Read the model definition and answer for the solid it produces. Units are mm, in the model's axes. Face numbers are marked on the shaded views. A direction names the side the tool comes from. Coordinates: 2 decimals unless noted, no trailing zeros. Loops run counter-clockwise (first coordinate to the right, second up) from the corner with the lowest first, then second, coordinate; pieces in that order, holes last. Notation, with made-up numbers: (63.25, 68.5) -> (77.25, 68.5) arc R28 ccw to (77.25, 86.5) -> close; hole circle Ø2 at (-35, 22.25). An arc over 180 degrees is marked (long way). Answer in a Markdown table with one row per item.
```python
from build123d import *

# Parameters (mm, degrees)
F0_W     = 30
F0_H     = 30
F1_DEPTH = 30
F2_SIZE  = 3.1
F3_R     = 10
F4_DEPTH = 32.5
F6_DEPTH = 1
F8_DEPTH = 1


with BuildPart() as f1:
    # F0 (on Top) → F1 (new body)
    with BuildSketch(Plane.XY):
        Rectangle(F0_W, F0_H)
    extrude(amount=F1_DEPTH)

    # F2
    f2_edges = [f1.edges().sort_by_distance(p)[0] for p in [
        (0, -15, 30),
        (15, 0, 30),
        (15, -15, 15),
        (-15, 0, 0),
        (0, 15, 0),
        (-15, 15, 15),
        (0, 15, 30),
        (15, 15, 15),
        (-15, -15, 15),
        (0, -15, 0),
        (15, 0, 0),
        (-15, 0, 30),
    ]]
    chamfer(f2_edges, length=F2_SIZE)

    # F3 (on Top) → F4 (join)
    with BuildSketch(Plane.XY):
        Circle(F3_R)
    extrude(amount=F4_DEPTH)

    # F5 (on face) → F6 (join)
    with BuildSketch(Plane.XZ.offset(15)):
        Polygon((-9.9, 26.9), (-9.9, 3.1), (-4.9, 3.1), align=None)
        Polygon((9.9, 3.1), (9.9, 26.9), (4.9, 26.9), align=None)
        Polygon((-7.9, 26.9), (-2.9, 3.1), (7.9, 3.1), (2.9, 26.9), align=None)
    extrude(amount=F6_DEPTH)

    # F7 (on face) → F8 (join)
    with BuildSketch(Plane(origin=(0, 15, 0), x_dir=(-1, 0, 0), z_dir=(0, 1, 0))):
        Polygon((-2.9, 26.9), (-7.9, 3.1), (2.9, 3.1), (7.9, 26.9), align=None)
        Polygon((9.9, 26.9), (4.9, 3.1), (9.9, 3.1), align=None)
        Polygon((-4.9, 26.9), (-9.9, 26.9), (-9.9, 3.1), align=None)
    extrude(amount=F8_DEPTH)


solid = f1.part
```
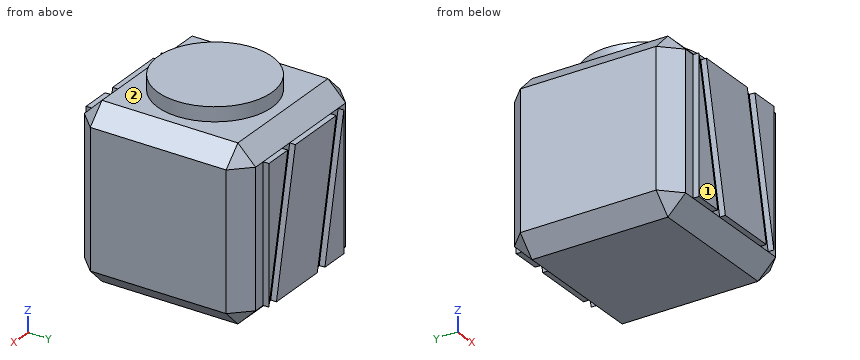
1. A cutting plane is placed at D-D on x = 6.75. Give the vertices of the cut face in (y, z).
A:
| item | result |
|---|---|
| outline | (-16, 3.1) -> (-15, 3.1) -> (-11.9, 0) -> (11.9, 0) -> (15, 3.1) -> (16, 3.1) -> (16, 8.57) -> (15, 8.57) -> (15, 18.09) -> (16, 18.09) -> (16, 26.9) -> (15, 26.9) -> (11.9, 30) -> (7.38, 30) -> (7.38, 32.5) -> (-7.38, 32.5) -> (-7.38, 30) -> (-11.9, 30) -> (-15, 26.9) -> (-16, 26.9) -> (-16, 18.09) -> (-15, 18.09) -> (-15, 8.57) -> (-16, 8.57) -> close |
2. A tool of negligible diameter and unlimited length cuts with its end or side. For the marked faces 1 and 2, from which of +Z, -Z, +X, -X, +Y, -Y can it reach the whole face along a straight path? Write none if from no direction.
A:
| item | result |
|---|---|
| face 1 | +Z, -Z, +X, -X, -Y |
| face 2 | +Z |
3. A cutting plane is placed at A-A on z = 28. Give the vertices of the cut face in (x, y), and give its area (3 significant figures).
A:
| item | result |
|---|---|
| outline | (-13.9, -11.9) -> (-11.9, -13.9) -> (11.9, -13.9) -> (13.9, -11.9) -> (13.9, 11.9) -> (11.9, 13.9) -> (-11.9, 13.9) -> (-13.9, 11.9) -> close |
| area | 765 mm2 |
4. Find the intervals of material crossed by probe 1 along Z at (x, y) = (-8, 7); probe 2 along Y at (x, z) = (-5.5, 13); probe 3 along Y at (x, z) = (-12, 13.5), in increasing order.
A:
| item | result |
|---|---|
| probe 1 | z = 0 to 30 |
| probe 2 | y = -15 to 15 |
| probe 3 | y = -14.9 to 14.9 |
5. A cutting plane is placed at C-C on x = 0. Give the vertices of the cut face in (y, z), and give its area (3 significant figures).
A:
| item | result |
|---|---|
| outline | (-16, 3.1) -> (-15, 3.1) -> (-11.9, 0) -> (11.9, 0) -> (15, 3.1) -> (16, 3.1) -> (16, 26.9) -> (15, 26.9) -> (11.9, 30) -> (10, 30) -> (10, 32.5) -> (-10, 32.5) -> (-10, 30) -> (-11.9, 30) -> (-15, 26.9) -> (-16, 26.9) -> close |
| area | 978 mm2 |
6. A cutting plane is placed at B-B on y = 0. Give the vertices of the cut face in (x, z).
A:
| item | result |
|---|---|
| outline | (-15, 3.1) -> (-11.9, 0) -> (11.9, 0) -> (15, 3.1) -> (15, 26.9) -> (11.9, 30) -> (10, 30) -> (10, 32.5) -> (-10, 32.5) -> (-10, 30) -> (-11.9, 30) -> (-15, 26.9) -> close |
7. Given pin 1 Ø0.8 at (x, y) = (-7, 15.5) entering from -Z; pin 2 Ø0.5 at (x, y) = (8, -15.5) entering from +Z; pin 3 Ø1.5 at (x, y) = (-6, 11) entering from +Z, each flat-ended and moving along its own axis, determine where each tip first touches the part or whether it passes through.
A:
| item | result |
|---|---|
| pin 1 | stops at z = 3.1 |
| pin 2 | stops at z = 26.9 |
| pin 3 | stops at z = 30 |
